from build123d import *

# Parameters (mm, degrees)
F1_DEPTH    = 18.4
F2_T        = -2
F3_DEPTH    = 0.2
F4_R        = 1.4
F4_W        = 2.9
F4_H        = 2.1
F4_W_2      = 2.2
F4_H_2      = 3.4
F5_DEPTH    = 12.8
F4_R_2      = 3.5
F6_DEPTH    = 15.5
F4_H_3      = 3.85
F7_DEPTH    = 9.5
F8_T4_DEPTH = 22.7734639037
F9_DEPTH    = 1.801
F11_DEPTH   = 1
F10_W       = 1.05
F10_H       = 5.5
F12_DEPTH   = 1.6
F10_H_2     = 10.9
F13_DEPTH   = 3


# Not quite as in the source:
# - a fillet or chamfer that OpenCascade refuses, or shapes differently, is made with other operations: its cross-section is extruded or revolved along the edge and cut away or added


with BuildPart() as f1:
    # F0 (on Top) → F1 (new body)
    with BuildSketch(Plane.XY):
        with BuildLine():
            Line((-22.95, -42.3), (22.95, -42.3))
            ThreePointArc((22.95, -42.3), (28.2533008589, -40.1033008589), (30.45, -34.8))
            Line((30.45, -34.8), (30.45, 34.8))
            ThreePointArc((30.45, 34.8), (28.2533008589, 40.1033008589), (22.95, 42.3))
            Line((22.95, 42.3), (-22.95, 42.3))
            ThreePointArc((-22.95, 42.3), (-28.2533008589, 40.1033008589), (-30.45, 34.8))
            Line((-30.45, 34.8), (-30.45, -34.8))
            ThreePointArc((-30.45, -34.8), (-28.2533008589, -40.1033008589), (-22.95, -42.3))
        make_face()
    extrude(amount=F1_DEPTH)

    # F2
    f2_openings = [f1.faces().sort_by_distance(p)[0] for p in [
        (0, 0, 18.4),
    ]]
    offset(amount=F2_T, openings=f2_openings)

    # F3 (cut): a face of the model
    f3_faces = [f1.faces().sort_by_distance(p)[0] for p in [
        (0, 0, 0),
    ]]
    extrude(f3_faces, amount=-F3_DEPTH, mode=Mode.SUBTRACT)

    # F4 (on face) → F5 (join)
    with BuildSketch(Plane.XY.offset(2)):
        with BuildLine():
            Line((24.45, 6.62), (28.45, 6.62))
            Line((28.45, 6.62), (28.45, 10.78))
            Line((28.45, 10.78), (24.45, 10.78))
            ThreePointArc((24.45, 10.78), (22.37, 8.7), (24.45, 6.62))
        make_face()
        with Locations((24.45, 8.7)):
            Circle(F4_R, mode=Mode.SUBTRACT)
        with BuildLine():
            ThreePointArc((-24.45, 6.62), (-22.37, 8.7), (-24.45, 10.78))
            Line((-24.45, 10.78), (-28.45, 10.78))
            Line((-28.45, 10.78), (-28.45, 6.62))
            Line((-28.45, 6.62), (-24.45, 6.62))
        make_face()
        with Locations((-24.45, 8.7)):
            Circle(F4_R, mode=Mode.SUBTRACT)
        with Locations((-27, 33.35)):
            Rectangle(F4_W, F4_H)
        with Locations((-6.35, 38.6)):
            Rectangle(F4_W_2, F4_H_2)
        with BuildLine():
            ThreePointArc((16.2853761426, 31.995), (16.16, 33.12), (16.2853761426, 34.245))
            Line((16.2853761426, 34.245), (13.45, 34.245))
            Line((13.45, 34.245), (13.45, 31.995))
            Line((13.45, 31.995), (16.2853761426, 31.995))
        make_face()
    extrude(amount=F5_DEPTH)

    # F4 (on face) → F6 (join)
    with BuildSketch(Plane.XY.offset(2)):
        with BuildLine():
            Line((22.95, 40.3), (21.27, 40.3))
            Line((21.27, 40.3), (21.27, 38.23))
            ThreePointArc((21.27, 38.23), (18.0791262952, 37.1112936499), (16.2853761426, 34.245))
            ThreePointArc((16.2853761426, 34.245), (16.16, 33.12), (16.2853761426, 31.995))
            ThreePointArc((16.2853761426, 31.995), (21.835982371, 28.0414407598), (26.38, 33.12))
            Line((26.38, 33.12), (28.45, 33.12))
            Line((28.45, 33.12), (28.45, 34.8))
            ThreePointArc((28.45, 34.8), (26.8390872965, 38.6890872965), (22.95, 40.3))
        make_face()
        with Locations((21.27, 33.12)):
            Circle(F4_R_2, mode=Mode.SUBTRACT)
        with Locations((24.45, 8.7)):
            Circle(F4_R)
        with Locations((-24.45, 8.7)):
            Circle(F4_R)
    extrude(amount=F6_DEPTH)

    # F4 (on face) → F7 (join)
    with BuildSketch(Plane.XY.offset(2)):
        with Locations((-6.35, 34.975)):
            Rectangle(F4_W_2, F4_H_3)
    extrude(amount=F7_DEPTH)

    # F8: chamfer of 4 on 1 edges, made by hand


with BuildPart() as f8_tool2:
    # F8_s3 → F8_t4 (new body)
    with BuildSketch(Plane.YZ.offset(-17.7367319519)):
        Polygon((37.05, 11.5), (33.05, 7.5), (33.05, 11.5), align=None)
    extrude(amount=F8_T4_DEPTH)

    split(bisect_by=Plane.XZ.offset(-36.9), keep=Keep.TOP)


with BuildPart() as f1_1:
    add(f1.part)

    # F8_t1: cut F8_tool2
    add(f8_tool2.part, mode=Mode.SUBTRACT)

    # F4 (on face) → F9 (cut, through all)
    with BuildSketch(Plane.XY.offset(2)):
        with Locations((21.27, 33.12)):
            Circle(F4_R_2)
    extrude(amount=-F9_DEPTH, mode=Mode.SUBTRACT)

    # F10 (on face) → F11 (join)
    with BuildSketch(Plane.XZ.offset(-40.3)):
        Polygon((-8.45, 2), (-7.45, 2), (-7.45, 14.8), (-5.25, 14.8), (-5.25, 18.4), (-8.45, 18.4), align=None)
    extrude(amount=F11_DEPTH)

    # F10 (on face) → F12 (join)
    with BuildSketch(Plane.XZ.offset(-40.3)):
        Polygon((-22.95, 2), (-10.55, 2), (-10.55, 7.5), (-16.075, 7.5), (-16.075, 11.5), (-18.475, 11.5), (-18.475, 7.5), (-22.95, 7.5), align=None)
        with Locations((-23.475, 4.75)):
            Rectangle(F10_W, F10_H)
    extrude(amount=F12_DEPTH)

    # F10 (on face) → F13 (cut, symmetric)
    with BuildSketch(Plane.XZ.offset(-40.3)):
        Polygon((-10.55, 7.5), (-10.55, 18.4), (-22.95, 18.4), (-22.95, 7.5), (-18.475, 7.5), (-18.475, 11.5), (-16.075, 11.5), (-16.075, 7.5), align=None)
        with Locations((-23.475, 12.95)):
            Rectangle(F10_W, F10_H_2)
    extrude(amount=F13_DEPTH, both=True, mode=Mode.SUBTRACT)


solid = f1_1.part
Could you check a few things on this model? Use its own coordinates, in mm. A direction names the side the tool comes from. Give positions to 0.01 mm unless a question says otherwise; leave off trailing zeros. Write each loop counter-clockwise with the first axis right and the second up, starting at its lowest first coordinate (ties: lowest second). Pieces come first, ordered by that corner, then holes. Notation, with made-up numbers: (44, 47) -> (101, 47) arc R27 ccw to (101, 68) -> close; hole circle Ø1 at (-30.5, 34). An arc over 180 degrees is marked (long way). Answer as CSV lines item,"result". Start each with the question number.
(1) If we section it at A-A, the plane y = 8.7: Write out the boundary of the cut face in (x, z).
(2) Please list where these lines run through material, in increasing order: line 1 (X direction, y = 18.5, z = 12.75); line 2 (Y direction, x = -10.5, z = 12); line 3 (Y direction, x = 22, z = 14).
(3) I'm going to push flat-ended pins straight in: pin 1 Ø4 at (y, z) = (40, 9) entering from +X; pin 2 Ø1.2 at (x, z) = (-27, 9) entering from +Y; pin 3 Ø1.2 at (x, y) = (26.5, 8) entering from +Z. Where does each tip first touch, or does it pass through?
(4) If we section it at C-C, the plane z = 10.5: Give the number of separate pieces and of enclosed holes in the cut face, and give its area (3 significant figures).
(5) Which directions (+Z, -Z, +X, -X, +Y, -Y) give clear straight access to the entire face, cutting with the end or side of a thin tool? Please do faces 1 (the face through (-24, 41, 13)), 2 (the face through (28.195, -40.161, 9.173)), 3 (the face through (26, 9, 14.8)).
(6) If we section it at B-B, the plane x = 6: Write out the boundary of the cut face in (y, z), and give its area (3 significant figures).
Answer list:
1,outline,"(-30.45, 0.2) -> (30.45, 0.2) -> (30.45, 18.4) -> (28.45, 18.4) -> (28.45, 14.8) -> (25.85, 14.8) -> (25.85, 17.5) -> (23.05, 17.5) -> (23.05, 14.8) -> (22.37, 14.8) -> (22.37, 2) -> (-22.37, 2) -> (-22.37, 14.8) -> (-23.05, 14.8) -> (-23.05, 17.5) -> (-25.85, 17.5) -> (-25.85, 14.8) -> (-28.45, 14.8) -> (-28.45, 18.4) -> (-30.45, 18.4) -> close"
2,line 1,"-30.45 to -28.45, 28.45 to 30.45"
2,line 2,"-42.3 to -40.3, 40.3 to 42.3"
2,line 3,"-42.3 to -40.3, 28.06 to 29.7, 36.54 to 42.3"
3,pin 1,"x = 29.73"
3,pin 2,"y = 41.46"
3,pin 3,"z = 14.8"
4,separate pieces,"2"
4,enclosed holes,"1"
4,area,"663 mm^2"
5,face 1,"+Z, +Y"
5,face 2,"+Z, -Z, +X, -Y"
5,face 3,"+Z"
6,outline,"(-42.3, 0.2) -> (42.3, 0.2) -> (42.3, 18.4) -> (40.3, 18.4) -> (40.3, 2) -> (-40.3, 2) -> (-40.3, 18.4) -> (-42.3, 18.4) -> close"
6,area,"218 mm^2"
